Geometry check sheet. Reference: the model listing, model coordinates, mm. Face numbers are marked on the shaded views. Give positions to 0.01 mm unless a question says otherwise; leave off trailing zeros. Loops run counter-clockwise (first coordinate to the right, second up) from the corner with the lowest first, then second, coordinate; pieces in that order, holes last.
1. Material ranges on L1, parallel to Y at x = -9.5, z = 6; L2, parallel to Y at x = -7.5, z = -8.5; L3, parallel to Y at x = 11.75, z = -2.5, recorded low to high.
2. Cross-section at A-A, the plane x = 0. Record the cut outline in (y, z), plus the area to 3 significant figures.
3. Release check for a two-part mould opening along Y. For the marked faces 1, 2, 3 and 4 record: +Y half, -Y half, draft (parallel to the pull), parting line (faces both ways), or undercut.
4. Cross-section at C-C, the plane y = 21.75. Record the cut outline in (x, z).
5. Cross-section at B-B, the plane y = 25.25. Record the cut outline in (x, z), plus the area to 3 significant figures.
6. Go/stop test with flat-tipped pins: pin 1 Ø3.5 at (x, y) = (-6.5, 19.5) entering from +Z; pin 2 Ø2.5 at (x, y) = (-6.5, 18) entering from -Z; pin 3 Ø2 at (x, z) = (9.5, 10) entering from -Y; pin 4 Ø1.5 at (y, z) = (22.5, 11) entering from +X. Record where each tip stops, or that it passes through.
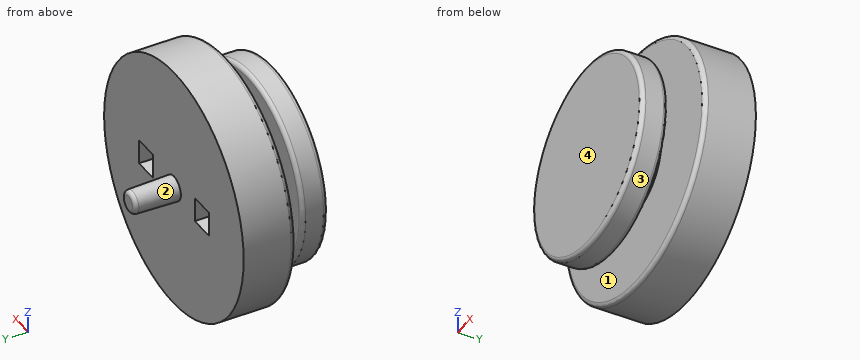
from build123d import *

# Parameters (mm, degrees)
SKETCH1_R           = 5.75
BOSS_EXTRUDE1_DEPTH = 15
SKETCH12_R          = 5.75
BOSS_EXTRUDE3_DEPTH = 2
SKETCH11_R          = 15
SKETCH11_W          = 3
SKETCH11_H          = 3
BOSS_EXTRUDE2_DEPTH = 4.25
SKETCH13_R          = 1.5
BOSS_EXTRUDE4_DEPTH = 5.5
BOSS_EXTRUDE4_TAPER = 1.5
FILLET2_R           = 0.5
BOSS_EXTRUDE5_START = -2
SKETCH11_2_R        = 15
BOSS_EXTRUDE5_DEPTH = 2
SKETCH14_R          = 11.75
BOSS_EXTRUDE6_DEPTH = 12.4
SKETCH14_2_R        = 11.75
CUT_EXTRUDE1_DEPTH  = 9.25
FILLET3_R           = 0.5


with BuildPart() as part:
    # Sketch1 → Boss-Extrude1 (new body)
    with BuildSketch(Plane(origin=(0, 0, 0), x_dir=(1, 0, 0), z_dir=(0, 1, 0))):
        with Locations(Location((0, 0, 0), (0, 0, 270))):
            Circle(SKETCH1_R)
    extrude(amount=BOSS_EXTRUDE1_DEPTH)

    # Sketch12 → Boss-Extrude3 (add)
    with BuildSketch(Plane(origin=(0, 15, 0), x_dir=(1, 0, 0), z_dir=(0, 1, 0))):
        with Locations(Location((0, 0, 0), (0, 0, 270))):
            Circle(SKETCH12_R)
    extrude(amount=BOSS_EXTRUDE3_DEPTH)

    # Sketch11 → Boss-Extrude2 (add)
    with BuildSketch(Plane(origin=(0, 17, 0), x_dir=(1, 0, 0), z_dir=(0, 1, 0))):
        with Locations(Location((0, 0, 0), (0, 0, 270))):
            Circle(SKETCH11_R)
        with Locations((-6, 0)):
            Rectangle(SKETCH11_W, SKETCH11_H, mode=Mode.SUBTRACT)
        with Locations((6, 0)):
            Rectangle(SKETCH11_W, SKETCH11_H, mode=Mode.SUBTRACT)
    extrude(amount=BOSS_EXTRUDE2_DEPTH)

    # Sketch13 → Boss-Extrude4 (add)
    with BuildSketch(Plane(origin=(0, 21.25, 0), x_dir=(1, 0, 0), z_dir=(0, 1, 0))):
        Circle(SKETCH13_R)
    extrude(amount=BOSS_EXTRUDE4_DEPTH, taper=BOSS_EXTRUDE4_TAPER)

    # Fillet2
    fillet2_edges = [part.edges().sort_by_distance(p)[0] for p in [
        (-1.355977431, 26.75, 0),
    ]]
    fillet(fillet2_edges, radius=FILLET2_R)

    # Sketch11<2> → Boss-Extrude5 (add)
    # profile 1 of 3: a face of its own
    with BuildSketch(Plane(origin=(0, 17, 0), x_dir=(1, 0, 0), z_dir=(0, 1, 0)).offset(BOSS_EXTRUDE5_START)):
        with Locations(Location((0, 0, 0), (0, 0, 270))):
            Circle(SKETCH11_2_R)
        with BuildLine():
            Line((-7.5, -1.5), (-7.5, 1.5))
            Line((-7.5, 1.5), (-5.550900828, 1.5))
            ThreePointArc((-5.550900828, 1.5), (0, 5.75), (5.550900828, 1.5))
            Line((5.550900828, 1.5), (7.5, 1.5))
            Line((7.5, 1.5), (7.5, -1.5))
            Line((7.5, -1.5), (5.550900828, -1.5))
            ThreePointArc((5.550900828, -1.5), (0, -5.75), (-5.550900828, -1.5))
            Line((-5.550900828, -1.5), (-7.5, -1.5))
        make_face(mode=Mode.SUBTRACT)
    # profile 2 of 3: a face of its own
    with BuildSketch(Plane(origin=(0, 17, 0), x_dir=(1, 0, 0), z_dir=(0, 1, 0)).offset(BOSS_EXTRUDE5_START)):
        with BuildLine():
            Line((7.5, 1.5), (5.550900828, 1.5))
            ThreePointArc((5.550900828, 1.5), (5.700007884, 0.756577901), (5.75, 0))
            ThreePointArc((5.75, 0), (5.700007884, -0.756577901), (5.550900828, -1.5))
            Line((5.550900828, -1.5), (7.5, -1.5))
            Line((7.5, -1.5), (7.5, 1.5))
        make_face()
    # profile 3 of 3: a face of its own
    with BuildSketch(Plane(origin=(0, 17, 0), x_dir=(1, 0, 0), z_dir=(0, 1, 0)).offset(BOSS_EXTRUDE5_START)):
        with BuildLine():
            Line((-5.550900828, 1.5), (-7.5, 1.5))
            Line((-7.5, 1.5), (-7.5, -1.5))
            Line((-7.5, -1.5), (-5.550900828, -1.5))
            ThreePointArc((-5.550900828, -1.5), (-5.75, 0), (-5.550900828, 1.5))
        make_face()
    extrude(amount=BOSS_EXTRUDE5_DEPTH)

    # Sketch14 → Boss-Extrude6 (add)
    with BuildSketch(Plane.XZ):
        with Locations(Location((0, 0, 0), (0, 0, 270))):
            Circle(SKETCH14_R)
    extrude(amount=-BOSS_EXTRUDE6_DEPTH)

    # Sketch14<2> → Cut-Extrude1 (cut)
    with BuildSketch(Plane.XZ):
        with Locations(Location((0, 0, 0), (0, 0, 270))):
            Circle(SKETCH14_2_R)
    extrude(amount=-CUT_EXTRUDE1_DEPTH, mode=Mode.SUBTRACT)

    # Fillet3
    fillet3_edges = [part.edges().sort_by_distance(p)[0] for p in [
        (0, 15, -15),
        (0, 12.4, 11.75),
        (0, 9.25, 11.75),
    ]]
    fillet(fillet3_edges, radius=FILLET3_R)


solid = part.part
Result:
1. L1: y = 9.25 to 12.4, 15 to 21.25
1. L2: y = 9.26 to 12.39, 15 to 21.25
1. L3: y = 15 to 21.25
2. outline: (9.25, -11.25) arc R0.5 ccw to (9.75, -11.75) - (11.9, -11.75) arc R0.5 ccw to (12.4, -11.25) - (12.4, -5.75) - (15, -5.75) - (15, -14.5) arc R0.5 ccw to (15.5, -15) - (21.25, -15) - (21.25, -1.5) - (26.26, -1.37) arc R0.5 ccw to (26.75, -0.87) - (26.75, 0.87) arc R0.5 ccw to (26.26, 1.37) - (21.25, 1.5) - (21.25, 15) - (15.5, 15) arc R0.5 ccw to (15, 14.5) - (15, 5.75) - (12.4, 5.75) - (12.4, 11.25) arc R0.5 ccw to (11.9, 11.75) - (9.75, 11.75) arc R0.5 ccw to (9.25, 11.25) - close
2. area: 307 mm2
3. face 1: undercut
3. face 2: +Y half
3. face 3: draft
3. face 4: -Y half
4. outline: circle Ø2.97 at (0, 0)
5. outline: circle Ø2.79 at (0, 0)
5. area: 6.12 mm2
6. pin 1: stops at z = 14.23
6. pin 2: stops at z = -14.05
6. pin 3: stops at y = 15
6. pin 4: passes through
